Autodesk Inventor part; units mm, degrees
ref_plane "YZ Plane" through (0, 0, 0) normal (1, 0, 0) x (0, 1, 0)
ref_plane "XZ Plane" through (0, 0, 0) normal (0, 1, 0) x (-1, 0, 0)
ref_plane "XY Plane" through (0, 0, 0) normal (0, 0, 1) x (1, 0, 0)
sketch "Sketch1" plane through (0, 0, 0) normal (0, 1, 0) x (-1, 0, 0)
  line L0 (0, 90) -> (-132, 90)
  line L1 (-132, 90) -> (-132, 0)
  line L2 (-132, 0) -> (0, 0)
  line L3 (0, 0) -> (0, 90)
  line L4 (0, 45) -> (-132, 45)
  line L5 (0, 65.5) -> (-20, 65.5)
  line L6 (-20, 65.5) -> (-20, 67)
  line L7 (-20, 67) -> (0, 67)
  line L8 (0, 67) -> (0, 65.5)
  line L9 (0, 23) -> (-20, 23)
  line L10 (-20, 23) -> (-20, 24.5)
  line L11 (-20, 24.5) -> (0, 24.5)
  line L12 (0, 24.5) -> (0, 23)
  circle A0 centre (-20, 65.5) radius 1.5
  circle A1 centre (-20, 24.5) radius 1.5
  dimension "d0" = 132
  dimension "d1" = 90
  dimension "d2" = 20
  dimension "d3" = 41
  dimension "d4" = 1.5
  dimension "d5" = 1.5
extrude "Extrusion1" add sketch "Sketch1" along normal blind 5 contours L3 L7 A0 L5 L4 L1 L0 | L4 L3 L11 A1 L9 L2 L1
sketch "Sketch2" plane through (0, 0, 90) normal (0, 0, 1) x (1, 0, 0)
  line L0 (0, 5) -> (132, 5)
  line L1 (22, 5) -> (19.75, 9.5)
  line L2 (19.75, 9.5) -> (29.25, 9.5)
  line L3 (29.25, 9.5) -> (27, 5)
  line L4 (24.5, 9.5) -> (24.5, 0)
  line L5 (132, 0) -> (0, 0)
  line L6 (72, 0) -> (72, 13)
  line L7 (132, 0) -> (132, 5)
  line L8 (122, 5) -> (124.25, 9.5)
  line L9 (124.25, 9.5) -> (114.75, 9.5)
  line L10 (114.75, 9.5) -> (117, 5)
  line L11 (117, 5) -> (122, 5)
  line L12 (132, 5) -> (0, 5)
  dimension "d8" = 9.5
  dimension "d10" = 22
  dimension "d11" = 5
  dimension "d15" = 4.5
  dimension "d90" = 60
extrude "Extrusion7" add sketch "Sketch2" against normal up to surface (90 mm away) contours L10 L9 L8 L0 | L0 L4 L2 L3 | L0 L1 L2 L4
sketch "Sketch3" plane through (132, 0, 90) normal (1, 0, 0) x (0, 0, -1)
  line L0 (0, 0) -> (90, 0)
  line L1 (0, 9.5) -> (90, 9.5)
  line L2 (90, 5) -> (0, 5)
  line L3 (22.5, 9.5) -> (67.5, 9.5)
  line L4 (67.5, 9.5) -> (67.5, 5)
  line L5 (67.5, 5) -> (22.5, 5)
  line L6 (22.5, 5) -> (22.5, 9.5)
  line L7 (0, 9.5) -> (0, 5)
  line L8 (90, 5) -> (90, 9.5)
  dimension "d93" = 45
  dimension "d94" = 22.5
  dimension "d95" = 22.5
extrude "Extrusion3" cut sketch "Sketch3" against normal blind 120 contours L1 L4 L2 L6
sketch "Sketch4" plane through (0, 5, 0) normal (0, 1, 0) x (1, 0, 0)
  line L0 (50, -27) -> (70, -27)
  line L1 (70, -27) -> (70, -63)
  line L2 (70, -63) -> (50, -63)
  line L3 (50, -63) -> (50, -66)
  line L4 (50, -66) -> (73, -66)
  line L5 (73, -66) -> (73, -24)
  line L6 (73, -24) -> (50, -24)
  line L7 (50, -24) -> (50, -27)
  line L8 (132, -90) -> (132, 0)
  line L9 (132, -45) -> (0, -45)
  line L10 (0, -24.5) -> (0, -65.5)
  point P0 (0, 0)
  dimension "d25" = 3
  dimension "d26" = 70
  dimension "d27" = 3
  dimension "d28" = 20
  dimension "d29" = 36
extrude "Extrusion4" add sketch "Sketch4" along normal blind 11
sketch "Sketch5" plane through (0, 16, 0) normal (0, 1, 0) x (1, 0, 0)
  line L0 (73, -24) -> (50, -24)
  line L1 (50, -63) -> (50, -66)
  line L2 (73, -24) -> (50, -24)
  line L3 (50, -24) -> (50, -66)
  line L4 (50, -66) -> (73, -66)
  line L5 (73, -66) -> (73, -24)
  point P0 (0, 0)
extrude "Extrusion5" add sketch "Sketch5" along normal blind 2
sketch "Sketch6" plane through (0, 0, 0) normal (0, -1, 0) x (1, 0, 0)
  line L0 (67.1453, 53) -> (87.1453, 53)
  line L1 (87.1453, 53) -> (87.1453, 37)
  line L2 (87.1453, 37) -> (67.1453, 37)
  line L3 (67.1453, 37) -> (67.1453, 53)
  line L4 (0, 90) -> (132, 90)
  line L5 (0, 24.5) -> (0, 65.5)
  line L6 (0, 45) -> (132, 45)
  line L7 (132, 90) -> (132, 0)
  line L8 (132, 0) -> (0, 0)
  line L9 (77.1453, 90) -> (77.1453, 0)
  line L10 (120, 85) -> (120, 62.5)
  line L11 (34, 85) -> (34, 62.5)
  line L12 (77.1453, 37) -> (77.1453, 32)
  line L13 (77.1453, 53) -> (77.1453, 58)
  line L14 (87.1453, 49) -> (86.1453, 49)
  dimension "d34" = 20
  dimension "d35" = 16
  dimension "d41" = 5
  dimension "d42" = 5
  dimension "d84" = 4
  dimension "d86" = 43.1454
  dimension "d88" = 43.1454
  dimension "d117" = 9
hole "Hole1" at (77.1453, 0, 32) at (86.1453, 0, 49) at (77.1453, 0, 58) direction (0, 1, 0) diameter 3 depth 8 tip angle 118
sketch "Sketch7" plane through (0, 0, 0) normal (0, -1, 0) x (1, 0, 0)
  line L0 (152, 71.65) -> (52, 71.65)
  line L1 (52, 71.65) -> (52, 18.35)
  line L2 (52, 18.35) -> (152, 18.35)
  line L3 (152, 18.35) -> (152, 71.65)
  line L4 (132, 90) -> (132, 0)
  line L5 (132, 45) -> (0, 45)
  line L6 (0, 24.5) -> (0, 65.5)
  line L7 (152, 25.95) -> (118.1, 25.95)
  line L8 (152, 53.85) -> (118.1, 53.85)
  line L9 (52, 69.05) -> (67.3, 69.05)
  line L10 (50, 66) -> (73, 66)
  point P0 (0, 0)
  dimension "d52" = 53.3
  dimension "d53" = 100
  dimension "d54" = 20
  dimension "d55" = 66.1
  dimension "d56" = 7.6
  dimension "d57" = 33.9
  dimension "d58" = 27.9
  dimension "d81" = 50.8
  dimension "d82" = 2.6
  dimension "d83" = 15.3
  dimension "d118" = 15.2
hole "Hole2" at (118.1, 0, 25.95) at (118.1, 0, 53.85) at (67.3, 0, 69.05) at (52, 0, 69.05) direction (0, 1, 0) diameter 3 depth 8 tip angle 118
chamfer "Chamfer1" distance 0.5 angle 45 6 edges at (61.5, 18, 24) (73, 18, 45) (61.5, 18, 66) (60, 16, 27) (70, 16, 45) (60, 16, 63)
fillet "Fillet1" radius 3 4 edges at (0, 2.5, 0) (0, 2.5, 90) (132, 2.5, 90) (132, 2.5, 0)
sketch "Sketch10" plane through (0, 0, 0) normal (0, -1, 0) x (1, 0, 0)
  line L0 (29.25, 90) -> (19.75, 90)
  line L1 (24.5, 0) -> (24.5, 90)
  line L2 (19.75, 90) -> (19.75, 67.5)
  line L3 (114.75, 90) -> (124.25, 90)
  line L4 (119.5, 90) -> (119.5, 0)
  line L5 (129, 0) -> (3, 0)
  line L6 (0, 80) -> (132, 80)
  line L7 (132, 87) -> (132, 3)
  line L8 (0, 10) -> (132, 10)
  line L9 (3, 90) -> (129, 90)
  line L10 (24.5, 80) -> (14.5, 80)
  line L11 (24.5, 80) -> (34.5, 80)
  line L12 (24.5, 10) -> (14.5, 10)
  line L13 (24.5, 10) -> (34.5, 10)
  line L14 (119.5, 10) -> (109.5, 10)
  line L15 (119.5, 80) -> (109.5, 80)
  point P0 (0, 0)
  dimension "d100" = 10
  dimension "d101" = 10
  dimension "d102" = 10
  dimension "d103" = 10
  dimension "d104" = 10
  dimension "d105" = 10
  dimension "d106" = 10
  dimension "d107" = 10
hole "Hole3" at (14.5, 0, 80) at (34.5, 0, 80) at (14.5, 0, 10) at (34.5, 0, 10) at (109.5, 0, 80) at (109.5, 0, 10) direction (0, 1, 0) diameter 3 depth 8 tip angle 118
sketch "Sketch11" plane through (0, 0, 0) normal (0, -1, 0) x (1, 0, 0)
  line L0 (129, 0) -> (3, 0)
  line L1 (31.1108, 0) -> (43.1108, 0) construction
  line L2 (43.1108, 0) -> (49, 21) construction
  line L3 (49, 21) -> (90.4829, 21) construction
  line L4 (90.4829, 21) -> (105.1108, 0) construction
  line L5 (105.1108, 0) -> (113.1108, 0) construction
  spline S0 degree 4 poles (31.1108, 0) (43.1108, 0) (49, 21) (90.4829, 21) (105.1108, 0) (113.1108, 0) knots 1 1 1 1 1 2 3 3 3 3 3
  line L6 (132, 87) -> (132, 3)
  line L7 (132, 45) -> (0, 45)
  line L8 (0, 24.5) -> (0, 65.5)
  line L9 (31.1108, 90) -> (43.1108, 90) construction
  line L10 (43.1108, 90) -> (49, 69) construction
  line L11 (49, 69) -> (90.4829, 69) construction
  line L12 (90.4829, 69) -> (105.1108, 90) construction
  line L13 (105.1108, 90) -> (113.1108, 90) construction
  spline S1 degree 4 poles (31.1108, 90) (43.1108, 90) (49, 69) (90.4829, 69) (105.1108, 90) (113.1108, 90) knots 1 1 1 1 1 2 3 3 3 3 3
  line L14 (3, 90) -> (129, 90)
  line L15 (27, 90) -> (117, 90)
  line L16 (31.1108, 90) -> (113.1108, 90)
  point P0 (0, 0)
extrude "Extrusion8" cut sketch "Sketch11" against normal blind 10
equation "\"d5\" = d4"
properties part number "one_part_body_V2"
Here's how the part is built. I have some questions about the finished solid (model axes, mm). A direction names the side the tool comes from. Coordinates: 2 decimals unless noted, no trailing zeros. Loops run counter-clockwise (first coordinate to the right, second up) from the corner with the lowest first, then second, coordinate; pieces in that order, holes last.
1. Imagine slicing it at B-B, the plane x = 14.5. Please give me the cut outline in (y, z).
2. Imagine slicing it at A-A, the plane z = 53.85. Please give me the cut outline in (x, y).
3. If we mould it in two halves opening along Z, with no side actions, what happens to faces 1 (the flat face through (9, 2, 65.5)), 2 (the flat face through (9, 2, 24.5)), 3 (the flat face through (132, 2, 46)), 4 (the flat face through (61, 11, 66))? For each: pulls with the +Z half, pulls with the -Z half, needs draft (parallel to the pull), parting line crosses it, or undercut.
4. For P1, Ø4, axis at y = 13.5, z = 47, coming from the +X side; P2, Ø4, axis at x = 34.5, z = 10, coming from the +Y side; P3, Ø3, axis at y = 8, z = 52, coming from the -X side; P4, Ø2.5, axis at x = 118.1, z = 53.85, coming from the +Y side, each with a flat end and sliding along its axis, tell me the tip position at first contact or that it passes through.
5. For faces 5 (the flat face through (25, 7, 22.5)), 6 (the cylindrical face through (108, 3, 10)), 7 (the flat face through (60, 16, 45)), 8 (the cylindrical face through (0.86, 2.54, 89.1)), 9 (the flat face through (123, 7, 11)), which set-ups out of +Z, -Z, +X, -X, +Y, -Y let a thin tool reach every point of the face, with its end or its side?
6. I need wall thicknesses on L1, parallel to Z at x = 11.5, y = 3.75; L2, parallel to X at y = 2.7, z = 69.05; L3, parallel to Z at x = 118.1, y = 2.65. Which ranges of each line are inside material? Lowest first, please.
7. Imagine slicing it at C-C, the plane z = 69.05. Please give me the cut outline in (x, y), and give its area (3 significant figures).
8. Imagine slicing it at D-D, the plane y = 11.5. Please give me the cut outline in (x, z), and give its area (3 significant figures).
Taken from the geometry:
1. outline: (0, 0) - (5, 0) - (5, 8.5) - (0, 8.5) - close; (0, 11.5) - (5, 11.5) - (5, 23) - (0, 23) - close; (0, 24.5) - (5, 24.5) - (5, 65.5) - (0, 65.5) - close; (0, 67) - (5, 67) - (5, 78.5) - (0, 78.5) - close; (0, 81.5) - (5, 81.5) - (5, 90) - (0, 90) - close
2. outline: (0, 0) - (116.6, 0) - (116.6, 5) - (73, 5) - (73, 17.5) - (72.5, 18) - (50, 18) - (50, 16) - (69.5, 16) - (70, 15.5) - (70, 5) - (0, 5) - close; (119.6, 0) - (132, 0) - (132, 5) - (119.6, 5) - close
3. face 1: undercut
3. face 2: undercut
3. face 3: needs draft
3. face 4: pulls with the +Z half
4. P1: stops at x = 73
4. P2: stops at y = 5
4. P3: stops at x = 70
4. P4: passes through
5. face 5: +X, -X, +Y
5. face 6: +Y, -Y
5. face 7: -X
5. face 8: +Z, -X, +Y, -Y
5. face 9: +Z, -Z, +X
6. L1: z = 0 to 23, 24.5 to 65.5, 67 to 90
6. L2: x = 0 to 50.5, 53.5 to 65.8, 68.8 to 132
6. L3: z = 0 to 24.45, 27.45 to 52.35, 55.35 to 90
7. outline: (0, 0) - (50.5, 0) - (50.5, 5) - (27, 5) - (29.25, 9.5) - (19.75, 9.5) - (22, 5) - (0, 5) - close; (53.5, 0) - (65.8, 0) - (65.8, 5) - (53.5, 5) - close; (68.8, 0) - (132, 0) - (132, 5) - (122, 5) - (124.25, 9.5) - (114.75, 9.5) - (117, 5) - (68.8, 5) - close
7. area: 695 mm2
8. outline: (50, 24) - (73, 24) - (73, 66) - (50, 66) - (50, 63) - (70, 63) - (70, 27) - (50, 27) - close
8. area: 246 mm2
